```python
from build123d import *

# Parameters (mm, degrees)
BOSS_EXTRUDE1_DEPTH = 42
CUT_EXTRUDE1_DEPTH  = 107.244079886


with BuildPart() as part:
    # Sketch2 → Boss-Extrude1 (new body)
    with BuildSketch(Plane(origin=(0, 0, 0), x_dir=(0, 0, -1), z_dir=(1, 0, 0))):
        Polygon((74.588748486, 0), (94.062768994, 0), (94.062768994, 3), (77.588748486, 3), (77.588748486, 26), (28.588748486, 26), (28.588748486, 10), (17.588748486, 10), (17.588748486, 7), (31.588748486, 7), (31.588748486, 23), (74.588748486, 23), align=None)
    extrude(amount=BOSS_EXTRUDE1_DEPTH)

    # Sketch3 → Cut-Extrude1 (cut, through all)
    with BuildSketch(Plane(origin=(0, 26, 0), x_dir=(1, 0, 0), z_dir=(0, 1, 0))):
        with BuildLine():
            Line((11, 17.588748486), (11, 44.782124623))
            ThreePointArc((11, 44.782124623), (21, 66.088748486), (31, 44.782124623))
            Line((31, 44.782124623), (31, 17.588748486))
            Line((31, 17.588748486), (11, 17.588748486))
        make_face()
    extrude(amount=-CUT_EXTRUDE1_DEPTH, mode=Mode.SUBTRACT)


solid = part.part
```
Could you check a few things on this model? Use its own coordinates, in mm. A direction names the side the tool comes from. Round coordinates to 2 decimals unless told otherwise and drop trailing zeros. Write each loop counter-clockwise with the first axis right and the second up, starting at its lowest first coordinate (ties: lowest second). Pieces come first, ordered by that corner, then holes.
(1) Suppose I cut it at C-C on z = -58. Write out the boundary of the cut face in (x, y).
Findings below:
outline: (0, 23) - (8.96, 23) - (8.96, 26) - (0, 26) - close; (33.04, 23) - (42, 23) - (42, 26) - (33.04, 26) - close
(2) Thinking about a two-plate mould opening in X: for faces 1 (the face through (0, 24, -58)), 2 (the face through (20.588, 24.521, -66.082)), 3 (the face through (36, 7, -24)), 4 (the face through (11, 17, -30)), which applies, +X half, -X half, draft (parallel to the pull), parting line (faces both ways), or undercut?
Findings below:
face 1: -X half
face 2: undercut
face 3: draft
face 4: undercut
(3) Suppose I cut it at A-A on y = 14.25. Write out the boundary of the cut face in (x, z), and give its area (3 significant figures).
Findings below:
outline: (0, -77.59) - (42, -77.59) - (42, -74.59) - (0, -74.59) - close; (0, -31.59) - (11, -31.59) - (11, -28.59) - (0, -28.59) - close; (31, -31.59) - (42, -31.59) - (42, -28.59) - (31, -28.59) - close
area: 192 mm2
(4) Suppose I cut it at B-B on x = 9. Write out the boundary of the cut face in (y, z).
Findings below:
outline: (0, -94.06) - (3, -94.06) - (3, -77.59) - (26, -77.59) - (26, -58.09) - (23, -58.09) - (23, -74.59) - (0, -74.59) - close; (7, -31.59) - (23, -31.59) - (23, -48.09) - (26, -48.09) - (26, -28.59) - (10, -28.59) - (10, -17.59) - (7, -17.59) - close
(5) Which directions (+Z, -Z, +X, -X, +Y, -Y) give clear straight access to the entire face, cutting with the end or side of a thin tool? Please do faces 5 (the face through (21, 23, -67)), 6 (the face through (21, 14, -77.589)), 7 (the face through (36, 10, -23)).
Findings below:
face 5: +X, -X, -Y
face 6: -Z, +X, -X, +Y
face 7: +Z, +X, -X, +Y
(6) If I drill on probe 1 along Z at (x, y) = (32, 12.5); probe 2 along Y at (x, z) = (2, -23); probe 3 along Z at (x, y) = (21, 24.85), over which ranges is the centre line in solid material (lowest first)?
Findings below:
probe 1: z = -77.59 to -74.59, -31.59 to -28.59
probe 2: y = 7 to 10
probe 3: z = -77.59 to -66.09
(7) For pin 1 (4 mm diameter, centred on x = 23.5, z = -82, fed in from +Y); pin 2 (5 mm diameter, centred on x = 9.5, y = 12.5, fed in from -Z); pin 3 (12 mm diameter, centred on x = 5.5, z = -26, fed in from -Y), each with a flat end and sliding along its axis, tell me the tip position at first contact or that it passes through.
Findings below:
pin 1: stops at y = 3
pin 2: stops at z = -77.59
pin 3: stops at y = 7
(8) Suppose I cut it at D-D on x = 21. Write out the boundary of the cut face in (y, z), and give its area (3 significant figures).
Findings below:
outline: (0, -94.06) - (3, -94.06) - (3, -77.59) - (26, -77.59) - (26, -66.09) - (23, -66.09) - (23, -74.59) - (0, -74.59) - close
area: 153 mm2
